Input: part model. Units: mm. Frame: model coordinates. A direction names the side the tool comes from. Give positions to 0.01 mm unless a question says otherwise; leave off trailing zeros. Order: outer loops, then holes, each group sorted by start corner. A loop starts at its lowest first (then second) coordinate and runs counter-clockwise, first axis right, second up. Notation, with made-up numbers: M 50,-37 L 70,-37 A16 ccw 70,-7 Z; hole C 75,32.5 d2. An arc over 180 degrees is marked long. Use a Markdown table: item, result.
from build123d import *

# Parameters (mm, degrees)
F1_DEPTH = 9.3
F2_R     = 7.4213549333
F2_R_2   = 3.1815358487
F2_R_3   = 2.3103538903
F2_R_4   = 2.3953978144
F2_R_5   = 2.4306675127
F3_DEPTH = 1.2


with BuildPart() as f1:
    # F0 (on Top) → F1 (new body)
    with BuildSketch(Plane.XY):
        with BuildLine():
            ThreePointArc((-18.3004729587, 25.7488646483), (-16.9307669757, 29.4600974462), (-16.9389080256, 33.4160141647))
            ThreePointArc((-16.9389080256, 33.4160141647), (-27.8122380676, 42.6489766388), (-38.8949178159, 33.6683802307))
            ThreePointArc((-38.8949178159, 33.6683802307), (-38.9054329765, 29.2141712974), (-37.1765067827, 25.1091862783))
            ThreePointArc((-37.1765067827, 25.1091862783), (-35.1477566437, 22.8641370486), (-32.5913859219, 21.2451738298))
            ThreePointArc((-32.5913859219, 21.2451738298), (-30.2580300956, 20.4751404155), (-27.8128294464, 20.2332837294))
            ThreePointArc((-27.8128294464, 20.2332837294), (-25.4265044225, 20.5189898006), (-23.1563369345, 21.3079857798))
            ThreePointArc((-23.1563369345, 21.3079857798), (-20.3943690235, 23.1631747639), (-18.3004729587, 25.7488646483))
        make_face()
        with BuildLine():
            ThreePointArc((-21.5058938379, 18.49241862), (-15.4174244879, 20.1391282026), (-18.3004729587, 25.7488646483))
            ThreePointArc((-18.3004729587, 25.7488646483), (-20.3943690235, 23.1631747639), (-23.1563369345, 21.3079857798))
            ThreePointArc((-23.1563369345, 21.3079857798), (-21.9745400177, 20.1092213147), (-21.5058938379, 18.49241862))
        make_face()
        with BuildLine():
            ThreePointArc((-32.5913859219, 21.2451738298), (-35.1477566437, 22.8641370486), (-37.1765067827, 25.1091862783))
            ThreePointArc((-37.1765067827, 25.1091862783), (-39.9197400879, 19.57935889), (-33.8508013782, 18.4513948615))
            ThreePointArc((-33.8508013782, 18.4513948615), (-33.5745375326, 20.0076143047), (-32.5913859219, 21.2451738298))
        make_face()
        with BuildLine():
            ThreePointArc((-21.5058938379, 18.49241862), (-22.6267961898, 19.7268785626), (-23.1563369345, 21.3079857798))
            ThreePointArc((-23.1563369345, 21.3079857798), (-25.4265044225, 20.5189898006), (-27.8128294464, 20.2332837294))
            ThreePointArc((-27.8128294464, 20.2332837294), (-27.4203125791, 18.5099777966), (-27.9959938241, 16.8389170756))
            ThreePointArc((-27.9959938241, 16.8389170756), (-24.0855301415, 15.0538762887), (-21.5058938379, 18.49241862))
        make_face()
        with BuildLine():
            ThreePointArc((-21.5058938379, 18.49241862), (-21.9745400177, 20.1092213147), (-23.1563369345, 21.3079857798))
            ThreePointArc((-23.1563369345, 21.3079857798), (-22.6267961898, 19.7268785626), (-21.5058938379, 18.49241862))
        make_face()
        with BuildLine():
            ThreePointArc((-27.8128294464, 20.2332837294), (-30.2580300956, 20.4751404155), (-32.5913859219, 21.2451738298))
            ThreePointArc((-32.5913859219, 21.2451738298), (-32.932636463, 19.7182499213), (-33.8508013782, 18.4513948615))
            ThreePointArc((-33.8508013782, 18.4513948615), (-31.4928658765, 15.5774517251), (-27.9959938241, 16.8389170756))
            ThreePointArc((-27.9959938241, 16.8389170756), (-28.3547938845, 18.5604036062), (-27.8128294464, 20.2332837294))
        make_face()
        with BuildLine():
            ThreePointArc((-33.8508013782, 18.4513948615), (-32.932636463, 19.7182499213), (-32.5913859219, 21.2451738298))
            ThreePointArc((-32.5913859219, 21.2451738298), (-33.5745375326, 20.0076143047), (-33.8508013782, 18.4513948615))
        make_face()
        with BuildLine():
            ThreePointArc((-27.9959938241, 16.8389170756), (-27.4203125791, 18.5099777966), (-27.8128294464, 20.2332837294))
            ThreePointArc((-27.8128294464, 20.2332837294), (-28.3547938845, 18.5604036062), (-27.9959938241, 16.8389170756))
        make_face()
    extrude(amount=F1_DEPTH)

    # F2 (on face) → F3 (join)
    with BuildSketch(Plane.XY.offset(9.3)):
        with Locations((-27.9406308089, 31.4787256965)):
            Circle(F2_R)
        with Locations((-36.4591698118, 21.3079857798)):
            Circle(F2_R_2)
        with Locations((-30.5455215275, 19.5178873837)):
            Circle(F2_R_3)
        with Locations((-24.4818478823, 19.4336697459)):
            Circle(F2_R_4)
        with Locations((-18.2497408241, 21.7075478286)):
            Circle(F2_R_5)
    extrude(amount=F3_DEPTH)


solid = f1.part
1) Mould query, pull axis Y, two halves, no side actions, for faces 1 (the face through (-28, 23, 9.3)), 2 (the face through (-27.596, 42.644, 4.585)), 3 (the face through (-31, 20, 10.5)). Classes: released by +Y, released by -Y, zero draft, split by the parting line, or undercut.
Response values:
| item | result |
|---|---|
| face 1 | undercut |
| face 2 | released by +Y |
| face 3 | zero draft |
2) Cut plane A-A on x = -30.5. Return loops of the section in (y, z), and give its area (3 significant figures).
Response values:
| item | result |
|---|---|
| outline | M 15.46,0 L 42.35,0 L 42.35,9.3 L 38.44,9.3 L 38.44,10.5 L 24.51,10.5 L 24.51,9.3 L 21.83,9.3 L 21.83,10.5 L 17.21,10.5 L 17.21,9.3 L 15.46,9.3 Z |
| area | 272 mm² |
3) Cut plane B-B on y = 34.5. Return loops of the section in (x, z), and give its area (3 significant figures).
Response values:
| item | result |
|---|---|
| outline | M -38.7,0 L -17.19,0 L -17.19,9.3 L -21.16,9.3 L -21.16,10.5 L -34.72,10.5 L -34.72,9.3 L -38.7,9.3 Z |
| area | 216 mm² |
4) Material intervals for line 1 (Z direction, x = -17.75, y = 30.5); line 2 (X direction, y = 31.25, z = 8.25); line 3 (X direction, y = 16.5, z = 5.75), sorted ascending. Write a range as from..to.
Response values:
| item | result |
|---|---|
| line 1 | z = 0..9.3 |
| line 2 | x = -39.12..-16.76 |
| line 3 | x = -33.01..-28.27, -27.8..-22.06 |
5) Cut plane D-D on x = -26.5. Return loops of the section in (y, z), and give its area (3 significant figures).
Response values:
| item | result |
|---|---|
| outline | M 15.33,0 L 42.56,0 L 42.56,9.3 L 38.76,9.3 L 38.76,10.5 L 24.2,10.5 L 24.2,9.3 L 20.72,9.3 L 20.72,10.5 L 18.14,10.5 L 18.14,9.3 L 15.33,9.3 Z |
| area | 274 mm² |
6) Reachability of faces 4 (the face through (-32.854, 19.619, 9.892)), 5 (the face through (-37, 21, 10.5)) from +Z, -Z, +X, -X, +Y, -Y: full face, straight path, thin tool, end or side. Return the list, or none.
Response values:
| item | result |
|---|---|
| face 4 | +Z |
| face 5 | +Z, +X, -X, +Y, -Y |
7) Cut plane C-C on z = 7.25. Return loops of the section in (x, y), and give its area (3 significant figures).
Response values:
| item | result |
|---|---|
| outline | M -38.89,33.67 A11.18 ccw -37.18,25.11 A3.87 ccw long -33.85,18.45 A3.22 ccw -28,16.84 A3.43 ccw -21.51,18.49 A4.06 ccw long -18.3,25.75 A11.18 ccw -16.94,33.42 A11.17 ccw Z |
| area | 531 mm² |
8) First-contact query: pin 1 Ø1.5 at (y, z) = (20, 8) entering from -X; pin 2 Ø5 at (x, z) = (-22, 5) entering from +Y; pin 3 Ø2 at (x, z) = (-30.5, 7.5) entering from -Y. Flat tips, straight axial feed; report the tip coordinate or a pass-through.
Response values:
| item | result |
|---|---|
| pin 1 | stops at x = -40.29 |
| pin 2 | stops at y = 42.11 |
| pin 3 | stops at y = 15.46 |
